from build123d import *

# Parameters (mm, degrees)
F0_R     = 34.0995
F1_DEPTH = 38.608
F3_R     = 36.1061
F4_DEPTH = 3.175
F6_R     = 36.1061
F7_DEPTH = 3.175


with BuildPart() as f1:
    # F0 (on Top) → F1 (new body)
    with BuildSketch(Plane.XY):
        with BuildLine():
            ThreePointArc((-164.9993838278, 120.7608555636), (0, 204.47), (164.9993838278, 120.7608555636))
            ThreePointArc((164.9993838278, 120.7608555636), (169.1054469037, 119.8617116159), (170.5054247616, 123.8250783438))
            Line((170.5054247616, 123.8250783438), (71.4788316492, 369.0016363528))
            ThreePointArc((71.4788316492, 369.0016363528), (0, 417.2204), (-71.4788316492, 369.0016363528))
            Line((-71.4788316492, 369.0016363528), (-170.5054247616, 123.8250783438))
            ThreePointArc((-170.5054247616, 123.8250783438), (-169.1054469037, 119.8617116159), (-164.9993838278, 120.7608555636))
        make_face()
        with Locations((0, 340.1314)):
            Circle(F0_R, mode=Mode.SUBTRACT)
    extrude(amount=F1_DEPTH)

    # F3 (on offset) → F4 (cut)
    with BuildSketch(Plane.XY.offset(32.258)):
        with Locations((0, 340.1314)):
            Circle(F3_R)
    extrude(amount=-F4_DEPTH, mode=Mode.SUBTRACT)

    # F6 (on offset) → F7 (cut)
    with BuildSketch(Plane.XY.offset(6.858)):
        with Locations((0, 340.1314)):
            Circle(F6_R)
    extrude(amount=-F7_DEPTH, mode=Mode.SUBTRACT)


solid = f1.part
Here's how the part is built. I have some questions about the finished solid (model axes, mm). A direction names the side the tool comes from. Coordinates: 2 decimals unless noted, no trailing zeros. Write each loop counter-clockwise with the first axis right and the second up, starting at its lowest first coordinate (ties: lowest second). Pieces come first, ordered by that corner, then holes.
1) If we section it at B-B (y = 364): List the corners of the cut face in (x, z) for me.
Filled in:
outline: (-73.5, 0) - (-24.35, 0) - (-24.35, 3.68) - (-27.09, 3.68) - (-27.09, 6.86) - (-24.35, 6.86) - (-24.35, 29.08) - (-27.09, 29.08) - (-27.09, 32.26) - (-24.35, 32.26) - (-24.35, 38.61) - (-73.5, 38.61) - close; (24.35, 0) - (73.5, 0) - (73.5, 38.61) - (24.35, 38.61) - (24.35, 32.26) - (27.09, 32.26) - (27.09, 29.08) - (24.35, 29.08) - (24.35, 6.86) - (27.09, 6.86) - (27.09, 3.68) - (24.35, 3.68) - close
2) If we section it at A-A (x = 0): List the corners of the cut face in (y, z) for me, plus the area to 3 significant figures.
Filled in:
outline: (204.47, 0) - (306.03, 0) - (306.03, 3.68) - (304.03, 3.68) - (304.03, 6.86) - (306.03, 6.86) - (306.03, 29.08) - (304.03, 29.08) - (304.03, 32.26) - (306.03, 32.26) - (306.03, 38.61) - (204.47, 38.61) - close; (374.23, 0) - (417.22, 0) - (417.22, 38.61) - (374.23, 38.61) - (374.23, 32.26) - (376.24, 32.26) - (376.24, 29.08) - (374.23, 29.08) - (374.23, 6.86) - (376.24, 6.86) - (376.24, 3.68) - (374.23, 3.68) - close
area: 5,560 mm2
3) If we section it at D-D (y = 398.5): List the corners of the cut face in (x, z) for me, plus the area to 3 significant figures.
Filled in:
outline: (-50.36, 0) - (50.36, 0) - (50.36, 38.61) - (-50.36, 38.61) - close
area: 3,890 mm2
4) Thinking about a two-plate mould opening in X: for faces 3 (the face through (-7.827, 304.884, 5.293)), 4 (the face through (121.685, 244.697, 19.034)), 5 (the face through (1.28, 417.21, 19.03)), which applies, +X half, -X half, draft (parallel to the pull), parting line (faces both ways), or undercut?
Filled in:
face 3: undercut
face 4: +X half
face 5: parting line
5) Which directions (+Z, -Z, +X, -X, +Y, -Y) give clear straight access to the entire face, cutting with the end or side of a thin tool? Please do faces 1 (the face through (27, 362, 6.858)), 2 (the face through (-2.688, 204.452, 19.034)).
Filled in:
face 1: none
face 2: +Z, -Z, -Y
6) I'm going to push flat-ended pins straight in: pin 1 (1.5 mm diameter, centred on x = 32.5, z = 30.5, fed in from +Y); pin 2 (8 mm diameter, centred on y = 252.5, z = 29, fed in from -X); pin 3 (2 mm diameter, centred on x = 71, z = 9.5, fed in from +Y). Where does each tip first touch, or does it pass through?
Filled in:
pin 1: stops at y = 410.38
pin 2: stops at x = -120.15
pin 3: stops at y = 372.42
7) If I drill on line 1 (Y direction, x = 32, z = 31.5); line 2 (X direction, y = 337.5, z = 21.5); line 3 (X direction, y = 147.5, z = 20.5), over which ranges is the centre line in solid material (lowest first)?
Filled in:
line 1: y = 201.95 to 323.41, 356.85 to 410.26
line 2: x = -84.2 to -34, 34 to 84.2
line 3: x = -160.94 to -141.6, 141.6 to 160.94
